Build history of the part. All positions in model axes, mm. Face numbers are marked on the shaded views. A direction names the side the tool comes from. Round coordinates to 2 decimals unless told otherwise and drop trailing zeros. Write each loop counter-clockwise with the first axis right and the second up, starting at its lowest first coordinate (ties: lowest second). Pieces come first, ordered by that corner, then holes. Notation, with made-up numbers: M -11.75,34 L 25.25,34 A14 cw 25.25,47 Z; hole C 11.25,34.5 d4. An arc over 180 degrees is marked long. One line per item, written item: value. Start each with the question number.
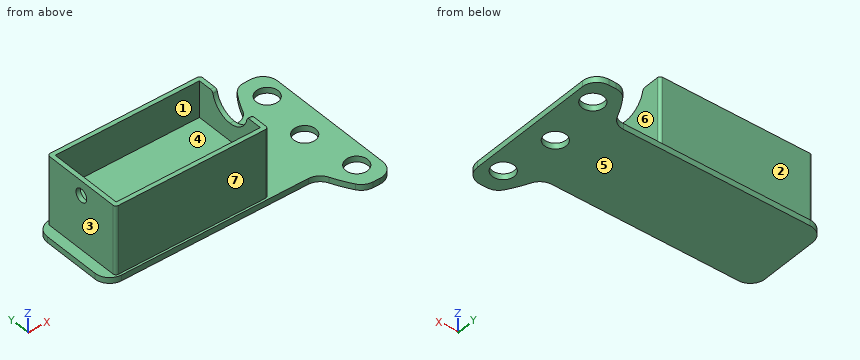
```python
from build123d import *

# Parameters (mm, degrees)
RESSALTO_EXTRUS_O1_DEPTH = 4
ESBO_O2_R                = 7.5
CORTE_EXTRUS_O1_DEPTH    = 10
ESBO_O3_W                = 145
ESBO_O3_H                = 60
RESSALTO_EXTRUS_O3_DEPTH = 4
RESSALTO_EXTRUS_O4_DEPTH = 47
CORTE_EXTRUS_O3_DEPTH    = 10
ESBO_O6_R                = 4.5
CORTE_EXTRUS_O4_DEPTH    = 9
FILETE1_R                = 10
FILETE3_R                = 10
FILETE4_R                = 2
ESBO_O7_W                = 99
ESBO_O7_H                = 51
RESSALTO_EXTRUS_O5_DEPTH = 22


with BuildPart() as part:
    # Esboço1 → Ressalto-extrusão1 (new body)
    with BuildSketch(Plane.XY):
        with BuildLine():
            Line((-72, -54), (-52, -54))
            Line((-52, -54), (-52, 54))
            Line((-52, 54), (-72, 54))
            ThreePointArc((-72, 54), (-90, 0), (-72, -54))
        make_face()
    extrude(amount=RESSALTO_EXTRUS_O1_DEPTH)

    # Esboço2 → Corte-extrusão1 (cut)
    with BuildSketch(Plane(origin=(0, 0, 0), x_dir=(-1, 0, 0), z_dir=(0, 0, -1))):
        with Locations((69.5, 0)):
            Circle(ESBO_O2_R)
        with Locations((64.5, -37.5)):
            Circle(ESBO_O2_R)
        with Locations((64.5, 37.5)):
            Circle(ESBO_O2_R)
    extrude(amount=-CORTE_EXTRUS_O1_DEPTH, mode=Mode.SUBTRACT)

    # Esboço3 → Ressalto-extrusão3 (add)
    with BuildSketch(Plane.XY):
        with Locations((-157.352813742, 0)):
            Rectangle(ESBO_O3_W, ESBO_O3_H)
    extrude(amount=RESSALTO_EXTRUS_O3_DEPTH)

    # Esboço4 → Ressalto-extrusão4 (add)
    with BuildSketch(Plane.XY.offset(4)):
        Polygon((-219.852813742, 0), (-222.852813742, 0), (-222.852813742, -28.5), (-117.852813742, -28.5), (-117.852813742, 0), (-120.852813742, 0), (-120.852813742, -25.5), (-219.852813742, -25.5), align=None)
        Polygon((-222.852813742, 28.5), (-222.852813742, 0), (-219.852813742, 0), (-219.852813742, 25.5), (-120.852813742, 25.5), (-120.852813742, 0), (-117.852813742, 0), (-117.852813742, 28.5), align=None)
    extrude(amount=RESSALTO_EXTRUS_O4_DEPTH)

    # Esboço5 → Corte-extrusão3 (cut)
    with BuildSketch(Plane(origin=(-117.852813742, 0, 0), x_dir=(0, 0, -1), z_dir=(1, 0, 0))):
        with BuildLine():
            Line((-51, 14.5), (-51, -14.5))
            ThreePointArc((-51, -14.5), (-41.725847678, -9.737171047), (-38, 0))
            ThreePointArc((-38, 0), (-41.725847678, 9.737171047), (-51, 14.5))
        make_face()
    extrude(amount=-CORTE_EXTRUS_O3_DEPTH, mode=Mode.SUBTRACT)

    # Esboço6 → Corte-extrusão4 (cut)
    with BuildSketch(Plane.ZY.offset(222.852813742)):
        with Locations((41, 0)):
            Circle(ESBO_O6_R)
    extrude(amount=-CORTE_EXTRUS_O4_DEPTH, mode=Mode.SUBTRACT)

    # Filete1
    filete1_edges = [part.edges().sort_by_distance(p)[0] for p in [
        (-229.852813742, 30, 2),
        (-229.852813742, -30, 2),
    ]]
    fillet(filete1_edges, radius=FILETE1_R)

    # Filete3
    filete3_edges = [part.edges().sort_by_distance(p)[0] for p in [
        (-84.852813742, 30, 2),
        (-84.852813742, -30, 2),
        (-72, 54, 2),
        (-52, 54, 2),
        (-52, -54, 2),
        (-72, -54, 2),
    ]]
    fillet(filete3_edges, radius=FILETE3_R)

    # Filete4
    filete4_edges = [part.edges().sort_by_distance(p)[0] for p in [
        (-117.852813742, -28.5, 27.5),
        (-117.852813742, 28.5, 27.5),
        (-222.852813742, 28.5, 27.5),
        (-222.852813742, -28.5, 27.5),
        (-119.352813742, 14.5, 51),
        (-119.352813742, -14.5, 51),
    ]]
    fillet(filete4_edges, radius=FILETE4_R)

    # Esboço7 → Ressalto-extrusão5 (add)
    with BuildSketch(Plane.XY.offset(4)):
        with Locations((-170.352813742, 0)):
            Rectangle(ESBO_O7_W, ESBO_O7_H)
    extrude(amount=RESSALTO_EXTRUS_O5_DEPTH)


solid = part.part
```
Item 1: Cut at C-C, the plane z = 6. Write the cut outline in (x, y).
Item 2: Cut at D-D, the plane z = 41. Write the cut outline in (x, y).
Item 3: Which spindle directions (+Z, -Z, +X, -X, +Y, -Y) get a long thin tool onto all of the face, cutting with end or side? Do the marked faces 4, 5, 6 and 7. Say none if no direction does.
Item 4: Drop flat-ended pins along their axis: pin 1 (4 mm diameter, centred on y = 13.5, z = 30.5, fed in from +X); pin 2 (7.5 mm diameter, centred on x = -162.5, z = 41, fed in from -Y); pin 3 (17 mm diameter, centred on x = -64.5, y = -37.5, fed in from +Z). Give the stop position or say it passes through.
Item 5: Two-plate mould, pull along X, no slides. Class the marked faces 1, 2 and 3: pulls with the +X half, pulls with the -X half, needs draft (parallel to the pull), parting line crosses it, or undercut.
Item 6: Drill centre lines: line 1 (Y direction, x = -221, z = 41); line 2 (X direction, y = -9, z = 32); line 3 (Y direction, x = -145.5, z = 34.5). Where is each one in solid material? Low to high.
Item 7: Cut at B-B, the plane x = -64.5. Write the cut outline in (y, z).
Item 8: Cut at A-A, the plane x = -161. Write the cut outline in (y, z).
Computed values:
1. outline: M -222.85,-26.5 A2 ccw -220.85,-28.5 L -119.85,-28.5 A2 ccw -117.85,-26.5 L -117.85,26.5 A2 ccw -119.85,28.5 L -220.85,28.5 A2 ccw -222.85,26.5 Z
2. outline: M -222.85,-26.5 A2 ccw -220.85,-28.5 L -119.85,-28.5 A2 ccw -117.85,-26.5 L -117.85,-8.86 L -120.85,-8.86 L -120.85,-25.5 L -219.85,-25.5 L -219.85,-4.5 L -222.85,-4.5 Z; M -222.85,4.5 L -219.85,4.5 L -219.85,25.5 L -120.85,25.5 L -120.85,8.86 L -117.85,8.86 L -117.85,26.5 A2 ccw -119.85,28.5 L -220.85,28.5 A2 ccw -222.85,26.5 Z
3. face 4: +Z
3. face 5: -Z, +X, -X, +Y, -Y
3. face 6: +Z, +X, +Y, -Y
3. face 7: +Z, +X, -X, -Y
4. pin 1: stops at x = -117.85
4. pin 2: stops at y = -28.5
4. pin 3: stops at z = 4
5. face 1: undercut
5. face 2: needs draft
5. face 3: pulls with the -X half
6. line 1: y = -28.49 to -4.5, 4.5 to 28.49
6. line 2: x = -222.85 to -219.85, -120.85 to -117.85
6. line 3: y = -28.5 to -25.5, 25.5 to 28.5
7. outline: M -54,0 L -45,0 L -45,4 L -54,4 Z; M -30,0 L -5.59,0 L -5.59,4 L -30,4 Z; M 5.59,0 L 30,0 L 30,4 L 5.59,4 Z; M 45,0 L 54,0 L 54,4 L 45,4 Z
8. outline: M -30,0 L 30,0 L 30,4 L 28.5,4 L 28.5,51 L 25.5,51 L 25.5,26 L -25.5,26 L -25.5,51 L -28.5,51 L -28.5,4 L -30,4 Z
